Input: part model. Units: mm. Frame: model coordinates. A direction names the side the tool comes from. Coordinates: 2 decimals unless noted, no trailing zeros. Write each loop counter-clockwise with the first axis right and the second up, starting at its lowest first coordinate (ties: lowest second). Pieces come first, ordered by that corner, then holes. Notation, with made-up numbers: (88, 42.25) -> (104, 42.25) arc R24 cw to (104, 74.25) -> close; hole circle Ø11 at (13.5, 12.5). An arc over 180 degrees is marked (long way). Use one line per item in the form item = value. Start each with the question number.
(1) Cut plane A-A on z = -83.3. State how many separate pieces and enclosed holes the cut face has, plus the area to 3 significant figures.
(2) Cut plane B-B on x = 0. Return the cut outline in (y, z), plus the area to 3 significant figures.
(3) Pull-direction query (Z, two-part tool) for faces 4 (the face through (12, 23, -140)), 5 (the face through (-39.53, 21.48, -105.31)), 6 (the face through (0.14, 24.24, -113.886)), 7 (the face through (16, 21.9, -95.6)); classes: released by +Z, released by -Z, zero draft, split by the parting line, or undercut.
(4) Ray query, line 1 along X through (y, z) = (22.55, -83.3); line 2 along X through (y, z) = (24.3, -115.5); line 3 along Z through (x, y) = (5.5, 22.8). Return the intervals inside material, ascending.
(5) First-contact query: pin 1 (1.5 mm diameter, centred on y = 21.5, z = -100, fed in from +X); pin 2 (2 mm diameter, centred on y = 22, z = -132.5, fed in from -X); pin 3 (2.5 mm diameter, centred on x = 14, y = 21.5, fed in from +Z). Flat tips, straight axial feed; report the tip coordinate or a pass-through.
(6) Set-up query: faces 1 (the face through (-34.34, 21.49, -142.22)), 2 (the face through (1.995, 21.922, -99.451)), 3 (the face through (2.364, 24.24, -118.092)). Return all of +Z, -Z, +X, -X, +Y, -Y with unobstructed straight access to the full face (end or side cutting, diameter ignored); none if empty.
```python
from build123d import *

# Parameters (mm, degrees)
BOSS_EXTRUDE1_START         = 10
SKETCH1_R                   = 1.15
BOSS_EXTRUDE1_DEPTH         = 76
SKETCH2_W                   = 6
SKETCH2_H                   = 16.4
CUT_EXTRUDE1_DEPTH          = 76
BOSS_EXTRUDE2_START         = -22
BOSS_EXTRUDE2_DEPTH         = 22
BOSS_EXTRUDE2_2_DEPTH       = 2
BOSS_EXTRUDE2_3_OUTLINE_W   = 6
BOSS_EXTRUDE2_3_OUTLINE_H   = 16
BOSS_EXTRUDE2_3_OUTLINE_W_2 = 5
BOSS_EXTRUDE2_3_OUTLINE_H_2 = 3
BOSS_EXTRUDE2_3_DEPTH       = 5
BOSS_EXTRUDE2_START_2       = -51.8
BOSS_EXTRUDE2_4_DEPTH       = 67
BOSS_EXTRUDE2_START_3       = -59
BOSS_EXTRUDE2_5_OUTLINE_R   = 1.15
BOSS_EXTRUDE2_5_DEPTH       = 78
CHAMFER1_SIZE               = 10
CHAMFER2_SIZE               = 4
CHAMFER3_SIZE               = 4
SKETCH4_W                   = 6
SKETCH4_H                   = 3.2
CUT_EXTRUDE2_DEPTH          = 17
CUT_EXTRUDE4_DEPTH          = 30
CUT_EXTRUDE4_DEPTH_BACK     = 41
SKETCH5_W                   = 96.095535807
SKETCH5_H                   = 97.903785136
SKETCH6_W                   = 65.908561939
SKETCH6_H                   = 2.295323053
CUT_EXTRUDE5_DEPTH          = 108
CUT_EXTRUDE6_DEPTH          = 108
SKETCH9_W                   = 18.2
SKETCH9_H                   = 56
CUT_EXTRUDE8_DEPTH          = 1.5
CUT_EXTRUDE9_DEPTH          = 13.5
CHAMFER4_SIZE               = 1.5
CHAMFER5_SIZE               = 1.5
CUT_EXTRUDE10_DEPTH         = 3.2
CUT_EXTRUDE11_DEPTH         = 3.2
CHAMFER6_SIZE               = 1.5
CUT_EXTRUDE12_DEPTH         = 26
SKETCH15_R                  = 4.5
CUT_EXTRUDE13_DEPTH         = 12


with BuildPart() as part:
    # Sketch1 → Boss-Extrude1 (new body)
    with BuildSketch(Plane(origin=(0, 0, -57.8), x_dir=(-1, 0, 0), z_dir=(0, 0, -1)).offset(BOSS_EXTRUDE1_START)):
        with BuildLine():
            Line((39, 25), (-18.2, 25))
            Line((-18.2, 25), (-18.2, 20))
            Line((-18.2, 20), (39, 20))
            ThreePointArc((39, 20), (41.5, 22.5), (39, 25))
        make_face()
        with Locations((39, 22.5)):
            Circle(SKETCH1_R, mode=Mode.SUBTRACT)
    extrude(amount=BOSS_EXTRUDE1_DEPTH)

    # Sketch2 → Cut-Extrude1 (cut)
    with BuildSketch(Plane(origin=(0, 25, 0), x_dir=(1, 0, 0), z_dir=(0, 1, 0))):
        with Locations((15.2, 105.8)):
            Rectangle(SKETCH2_W, SKETCH2_H)
    extrude(amount=-CUT_EXTRUDE1_DEPTH, mode=Mode.SUBTRACT)

    # Chamfer1
    chamfer1_edges = [part.edges().sort_by_distance(p)[0] for p in [
        (18.2, 22.5, -143.8),
        (18.2, 22.5, -67.8),
    ]]
    chamfer(chamfer1_edges, length=CHAMFER1_SIZE)

    # Chamfer2
    chamfer2_edges = [part.edges().sort_by_distance(p)[0] for p in [
        (18.2, 25, -87.7),
        (18.2, 25, -123.9),
    ]]
    chamfer(chamfer2_edges, length=CHAMFER2_SIZE)

    # Sketch4 → Cut-Extrude2 (cut)
    with BuildSketch(Plane(origin=(0, 25, 0), x_dir=(1, 0, 0), z_dir=(0, 1, 0))):
        with Locations((-38.5, 69.4)):
            Rectangle(SKETCH4_W, SKETCH4_H)
        with Locations((-38.5, 142.2)):
            Rectangle(SKETCH4_W, SKETCH4_H)
    extrude(amount=-CUT_EXTRUDE2_DEPTH, mode=Mode.SUBTRACT)

    # Sketch6 → Cut-Extrude5 (cut)
    with BuildSketch(Plane(origin=(0, 0, -143.8), x_dir=(-1, 0, 0), z_dir=(0, 0, -1))):
        with Locations((13.043955502, 19.152338474)):
            Rectangle(SKETCH6_W, SKETCH6_H)
    extrude(amount=-CUT_EXTRUDE5_DEPTH, mode=Mode.SUBTRACT)

    # Sketch7 → Cut-Extrude6 (cut)
    with BuildSketch(Plane(origin=(0, 0, -140.6), x_dir=(-1, 0, 0), z_dir=(0, 0, -1))):
        with BuildLine():
            Line((39, 24.7), (39, 27.795668708))
            Line((39, 27.795668708), (44.096773439, 22.698895269))
            Line((44.096773439, 22.698895269), (43.273657472, 20.3))
            Line((43.273657472, 20.3), (39, 20.3))
            ThreePointArc((39, 20.3), (41.2, 22.5), (39, 24.7))
        make_face()
    extrude(amount=-CUT_EXTRUDE6_DEPTH, mode=Mode.SUBTRACT)

    # Sketch9 → Cut-Extrude8 (cut)
    with BuildSketch(Plane(origin=(0, 25, 0), x_dir=(1, 0, 0), z_dir=(0, 1, 0))):
        with Locations((-19.9, 105.8)):
            Rectangle(SKETCH9_W, SKETCH9_H)
    extrude(amount=-CUT_EXTRUDE8_DEPTH, mode=Mode.SUBTRACT)

    # Sketch11 → Cut-Extrude9 (cut)
    with BuildSketch(Plane(origin=(0, 25, 0), x_dir=(1, 0, 0), z_dir=(0, 1, 0))):
        with BuildLine():
            Line((-3.382273892, 102.55565443), (7.524013646, 96.258906385))
            ThreePointArc((7.524013646, 96.258906385), (8.123454363, 94.021763172), (5.886311151, 93.422322455))
            Line((5.886311151, 93.422322455), (-5.019976387, 99.719070501))
            ThreePointArc((-5.019976387, 99.719070501), (-5.619417104, 101.956213713), (-3.382273892, 102.55565443))
        make_face()
        with BuildLine():
            Line((-3.382273892, 111.55565443), (7.524013646, 105.258906385))
            ThreePointArc((7.524013646, 105.258906385), (8.123454363, 103.021763172), (5.886311151, 102.422322455))
            Line((5.886311151, 102.422322455), (-5.019976387, 108.719070501))
            ThreePointArc((-5.019976387, 108.719070501), (-5.619417104, 110.956213713), (-3.382273892, 111.55565443))
        make_face()
        with BuildLine():
            Line((-3.382273892, 120.55565443), (7.524013646, 114.258906385))
            ThreePointArc((7.524013646, 114.258906385), (8.123454363, 112.021763172), (5.886311151, 111.422322455))
            Line((5.886311151, 111.422322455), (-5.019976387, 117.719070501))
            ThreePointArc((-5.019976387, 117.719070501), (-5.619417104, 119.956213713), (-3.382273892, 120.55565443))
        make_face()
    extrude(amount=-CUT_EXTRUDE9_DEPTH, mode=Mode.SUBTRACT)

    # Chamfer4
    chamfer4_edges = [part.edges().sort_by_distance(p)[0] for p in [
        (-19.9, 23.5, -133.8),
        (-10.8, 23.5, -105.8),
        (-19.9, 23.5, -77.8),
        (-29, 23.5, -105.8),
    ]]
    chamfer(chamfer4_edges, length=CHAMFER4_SIZE - 0.0001)  # a hair under: the kernel refuses the full size

    # Chamfer5
    chamfer5_edges = [part.edges().sort_by_distance(p)[0] for p in [
        (-5.619417104, 25, -110.956213713),
        (0.433167382, 25, -105.570696478),
        (8.123454363, 25, -103.021763172),
        (2.070869877, 25, -108.407280407),
        (-5.619417104, 25, -119.956213713),
        (0.433167382, 25, -114.570696478),
        (8.123454363, 25, -112.021763172),
        (2.070869877, 25, -117.407280407),
        (-5.619417104, 25, -101.956213713),
        (0.433167382, 25, -96.570696478),
        (8.123454363, 25, -94.021763172),
        (2.070869877, 25, -99.407280407),
    ]]
    chamfer(chamfer5_edges, length=CHAMFER5_SIZE)

    # Sketch12 → Cut-Extrude10 (cut)
    with BuildSketch(Plane(origin=(0, 0, -143.8), x_dir=(-1, 0, 0), z_dir=(0, 0, -1))):
        Polygon((35.5, 22.65), (33.15, 20.3), (34.627405096, 18.349875441), (37.777251213, 19.324937721), align=None)
    extrude(amount=-CUT_EXTRUDE10_DEPTH, mode=Mode.SUBTRACT)

    # Sketch13 → Cut-Extrude11 (cut)
    with BuildSketch(Plane.XY.offset(-67.8)):
        Polygon((-35.5, 22.65), (-33.15, 20.3), (-32.556705416, 17.347754732), (-36.536239956, 18.083750154), align=None)
    extrude(amount=-CUT_EXTRUDE11_DEPTH, mode=Mode.SUBTRACT)

    # Chamfer6
    chamfer6_edges = [part.edges().sort_by_distance(p)[0] for p in [
        (-35.5, 25, -69.4),
        (-35.5, 25, -142.2),
    ]]
    chamfer(chamfer6_edges, length=CHAMFER6_SIZE)

    # Sketch14 → Cut-Extrude12 (cut)
    with BuildSketch(Plane.XZ.offset(-20.3)):
        Polygon((18.2, -97.8), (14.7, -94.3), (14.7, -71.715249411), (21.506629366, -77.723703215), (19.139662716, -97.460563588), align=None)
    extrude(amount=-CUT_EXTRUDE12_DEPTH, mode=Mode.SUBTRACT)

    # Sketch15 → Cut-Extrude13 (cut)
    with BuildSketch(Plane.XZ.offset(-20.3)):
        with Locations(Location((0, -83.3, 0), (0, 0, 270))):
            Circle(SKETCH15_R)
    extrude(amount=-CUT_EXTRUDE13_DEPTH, mode=Mode.SUBTRACT)


with BuildPart() as body_2:
    # Boss-Extrude2: read off the stored shape, not the designer's step
    # Boss-Extrude2 outline → Boss-Extrude2 (new body)
    with BuildSketch(Plane(origin=(0, 20, 0), x_dir=(1, 0, 0), z_dir=(0, 1, 0)).offset(BOSS_EXTRUDE2_START)):
        Polygon((18.2, 47.8), (8.2, 57.8), (-41.5, 57.8), (-41.5, -18.2), (8.2, -18.2), (18.2, -8.2), align=None)
        with BuildLine():
            Line((-20, -15.2), (-38.5, -15.2))
            Line((-38.5, -15.2), (-38.5, 54.8))
            Line((-38.5, 54.8), (1.49684114, 54.8))
            Line((1.49684114, 54.8), (1.49684114, 39.499999909))
            Line((1.49684114, 39.499999909), (11.34684114, 39.499999909))
            Line((11.34684114, 39.499999909), (11.34684114, 10.113812147))
            ThreePointArc((11.34684114, 10.113812147), (0.0047491, -15.199999258), (-11.35315886, 10.10671974))
            Line((-11.35315886, 10.10671974), (-11.35315886, 39.499999909))
            Line((-11.35315886, 39.499999909), (-1.50315886, 39.499999909))
            Line((-1.50315886, 39.499999909), (-1.50315886, 51.8))
            Line((-1.50315886, 51.8), (-20, 51.8))
            Line((-20, 51.8), (-20, -15.2))
        make_face(mode=Mode.SUBTRACT)
    extrude(amount=BOSS_EXTRUDE2_DEPTH)

    # Boss-Extrude2 2 outline → Boss-Extrude2 2 (add)
    with BuildSketch(Plane(origin=(0, 20, 0), x_dir=(1, 0, 0), z_dir=(0, 1, 0)).offset(BOSS_EXTRUDE2_START)):
        with BuildLine():
            Line((1.49684114, 54.8), (-38.5, 54.8))
            Line((-38.5, 54.8), (-38.5, -15.2))
            Line((-38.5, -15.2), (-20, -15.2))
            Line((-20, -15.2), (-20, 51.8))
            Line((-20, 51.8), (-1.50315886, 51.8))
            Line((-1.50315886, 51.8), (-1.50315886, 39.499999909))
            Line((-1.50315886, 39.499999909), (-11.35315886, 39.499999909))
            Line((-11.35315886, 39.499999909), (-11.35315886, 10.10671974))
            ThreePointArc((-11.35315886, 10.10671974), (0.0047491, -15.199999258), (11.34684114, 10.113812147))
            Line((11.34684114, 10.113812147), (11.34684114, 39.499999909))
            Line((11.34684114, 39.499999909), (1.49684114, 39.499999909))
            Line((1.49684114, 39.499999909), (1.49684114, 54.8))
        make_face()
    extrude(amount=BOSS_EXTRUDE2_2_DEPTH)

    # Boss-Extrude2 3 outline → Boss-Extrude2 3 (add)
    with BuildSketch(Plane(origin=(0, 20, 0), x_dir=(1, 0, 0), z_dir=(0, 1, 0))):
        with Locations((15.2, 19.8)):
            Rectangle(BOSS_EXTRUDE2_3_OUTLINE_W, BOSS_EXTRUDE2_3_OUTLINE_H)
        with Locations((-39, 56.3)):
            Rectangle(BOSS_EXTRUDE2_3_OUTLINE_W_2, BOSS_EXTRUDE2_3_OUTLINE_H_2)
        with Locations((-39, -16.7)):
            Rectangle(BOSS_EXTRUDE2_3_OUTLINE_W_2, BOSS_EXTRUDE2_3_OUTLINE_H_2)
    extrude(amount=BOSS_EXTRUDE2_3_DEPTH)

    # Boss-Extrude2 4 outline → Boss-Extrude2 4 (cut)
    with BuildSketch(Plane.XY.offset(BOSS_EXTRUDE2_START_2)):
        Polygon((-20, 15.5), (-15.5, 20), (-20, 20), align=None)
    extrude(amount=BOSS_EXTRUDE2_4_DEPTH, mode=Mode.SUBTRACT)

    # Boss-Extrude2 5 outline → Boss-Extrude2 5 (cut)
    with BuildSketch(Plane.XY.offset(BOSS_EXTRUDE2_START_3)):
        with BuildLine():
            ThreePointArc((-41.5, 23), (-40.914213562, 24.414213562), (-39.5, 25))
            Line((-39.5, 25), (-41.5, 25))
            Line((-41.5, 25), (-41.5, 23))
        make_face()
        with BuildLine():
            ThreePointArc((-38.5, 25), (-37.085786438, 24.414213562), (-36.5, 23))
            Line((-36.5, 23), (-36.5, 25))
            Line((-36.5, 25), (-38.5, 25))
        make_face()
        with Locations((-39, 22.5)):
            Circle(BOSS_EXTRUDE2_5_OUTLINE_R)
    extrude(amount=BOSS_EXTRUDE2_5_DEPTH, mode=Mode.SUBTRACT)

    # Chamfer3
    chamfer3_edges = [body_2.edges().sort_by_distance(p)[0] for p in [
        (18.2, 25, -19.8),
    ]]
    chamfer(chamfer3_edges, length=CHAMFER3_SIZE)

    # Sketch5 → Cut-Extrude4 (cut, two sides: drawn at the far end of the back side and taken through both)
    with BuildSketch(Plane(origin=(0, 25, 0), x_dir=(1, 0, 0), z_dir=(0, 1, 0)).offset(-CUT_EXTRUDE4_DEPTH_BACK)):
        with Locations((-8.937626006, 13.848107432)):
            Rectangle(SKETCH5_W, SKETCH5_H)
    extrude(amount=CUT_EXTRUDE4_DEPTH + CUT_EXTRUDE4_DEPTH_BACK, mode=Mode.SUBTRACT)


solid = part.part
```
Values:
q1.separate_pieces = 2
q1.enclosed_holes = 1
q1.area = 188 mm2
q2.outline = (20.3, -143.8) -> (25, -143.8) -> (25, -120.33) -> (23.5, -118.6) -> (20.3, -118.6) -> close; (20.3, -114.82) -> (23.5, -114.82) -> (25, -113.09) -> (25, -111.33) -> (23.5, -109.6) -> (20.3, -109.6) -> close; (20.3, -105.82) -> (23.5, -105.82) -> (25, -104.09) -> (25, -102.33) -> (23.5, -100.6) -> (20.3, -100.6) -> close; (20.3, -96.82) -> (23.5, -96.82) -> (25, -95.09) -> (25, -87.8) -> (20.3, -87.8) -> close; (20.3, -78.8) -> (25, -78.8) -> (25, -67.8) -> (20.3, -67.8) -> close
q2.area = 254 mm2
q3.face_4 = released by -Z
q3.face_5 = zero draft
q3.face_6 = undercut
q3.face_7 = released by +Z
q4.line_1 = -41.2 to -40.15, -37.85 to -4.5, 4.5 to 14.7
q4.line_2 = -40.26 to -28.3, -11.5 to -2.78, 6.97 to 14.9
q4.line_3 = -143.8 to -115.43, -111.65 to -106.43, -102.65 to -97.43, -93.65 to -67.8
q5.pin_1 = 12.2
q5.pin_2 = -41.2
q5.pin_3 = -72.35
q6.face_1 = -Z, -X, -Y
q6.face_2 = +Y, -Y
q6.face_3 = +Y
